from build123d import *

# Parameters (mm, degrees)
SKETCH1_W                    = 1415
SKETCH1_H                    = 88
BASE_FLANGE1_DEPTH           = 4
EDGE_FLANGE1_STRIP_W         = 28
EDGE_FLANGE1_STRIP_H         = 4
EDGE_FLANGE1_STRIP_CUT_DEPTH = 1415
EDGE_FLANGE1_DEPTH           = 1415
EDGE_FLANGE2_STRIP_W         = 28
EDGE_FLANGE2_STRIP_H         = 4
EDGE_FLANGE2_STRIP_CUT_DEPTH = 1415
EDGE_FLANGE2_DEPTH           = 1415
CUT_EXTRUDE1_DEPTH           = 871.900176512
CUT_EXTRUDE1_DEPTH_BACK      = 871.900176512
SKETCH12_R                   = 11
CUT_EXTRUDE2_DEPTH           = 872.093059006
SKETCH16_R                   = 5
CUT_EXTRUDE4_DEPTH           = 10


# Sheet-metal steps are written as plain solids
with BuildPart() as part:
    # Sketch1 → Base-Flange1 (new body)
    with BuildSketch(Plane.XY):
        with Locations((-158.018987342, 44)):
            Rectangle(SKETCH1_W, SKETCH1_H)
    extrude(amount=-BASE_FLANGE1_DEPTH)

    # Edge-Flange1 strip (across the edge) → Edge-Flange1 strip cut (cut)
    with BuildSketch(Plane(origin=(549.481012658, 88, 0), x_dir=(0, -1, 0), z_dir=(-1, 0, 0))):
        with Locations((-4, -2)):
            Rectangle(EDGE_FLANGE1_STRIP_W, EDGE_FLANGE1_STRIP_H)
    extrude(amount=EDGE_FLANGE1_STRIP_CUT_DEPTH, mode=Mode.SUBTRACT)

    # Edge-Flange1 section (across the edge) → Edge-Flange1 (add)
    with BuildSketch(Plane(origin=(549.481012658, 88, 0), x_dir=(0, -1, 0), z_dir=(-1, 0, 0))):
        with BuildLine():
            Line((0, 6), (0, 40))
            Line((0, 40), (4, 40))
            Line((4, 40), (4, 6))
            ThreePointArc((4, 6), (5.757359313, 1.757359313), (10, 0))
            Line((10, 0), (10, -4))
            ThreePointArc((10, -4), (2.928932188, -1.071067812), (0, 6))
        make_face()
    extrude(amount=EDGE_FLANGE1_DEPTH)

    # Edge-Flange2 strip (across the edge) → Edge-Flange2 strip cut (cut)
    with BuildSketch(Plane.YZ.offset(-865.518987342)):
        with Locations((-4, -2)):
            Rectangle(EDGE_FLANGE2_STRIP_W, EDGE_FLANGE2_STRIP_H)
    extrude(amount=EDGE_FLANGE2_STRIP_CUT_DEPTH, mode=Mode.SUBTRACT)

    # Edge-Flange2 section (across the edge) → Edge-Flange2 (add)
    with BuildSketch(Plane.YZ.offset(-865.518987342)):
        with BuildLine():
            Line((0, 6), (0, 40))
            Line((0, 40), (4, 40))
            Line((4, 40), (4, 6))
            ThreePointArc((4, 6), (5.757359313, 1.757359313), (10, 0))
            Line((10, 0), (10, -4))
            ThreePointArc((10, -4), (2.928932188, -1.071067812), (0, 6))
        make_face()
    extrude(amount=EDGE_FLANGE2_DEPTH)

    # Sketch12 → Cut-Extrude1 (cut, two sides: drawn at the far end of the back side and taken through both)
    with BuildSketch(Plane.XZ.offset(-CUT_EXTRUDE1_DEPTH_BACK)):
        with Locations(Location((529.481012658, 20, 0), (0, 0, 270))):
            Circle(SKETCH12_R)
        with Locations(Location((449.481012658, 20, 0), (0, 0, 270))):
            Circle(SKETCH12_R)
    extrude(amount=CUT_EXTRUDE1_DEPTH + CUT_EXTRUDE1_DEPTH_BACK, mode=Mode.SUBTRACT)

    # Sketch13 → Cut-Extrude2 (cut, through all)
    with BuildSketch(Plane(origin=(0, 0, -4), x_dir=(-1, 0, 0), z_dir=(0, 0, -1))):
        with BuildLine():
            Line((850.518987342, 15), (830.518987342, 15))
            ThreePointArc((830.518987342, 15), (825.518987342, 20), (830.518987342, 25))
            Line((830.518987342, 25), (850.518987342, 25))
            ThreePointArc((850.518987342, 25), (855.518987342, 20), (850.518987342, 15))
        make_face()
        with BuildLine():
            Line((750.518987342, 15), (730.518987342, 15))
            ThreePointArc((730.518987342, 15), (725.518987342, 20), (730.518987342, 25))
            Line((730.518987342, 25), (750.518987342, 25))
            ThreePointArc((750.518987342, 25), (755.518987342, 20), (750.518987342, 15))
        make_face()
    extrude(amount=-CUT_EXTRUDE2_DEPTH, mode=Mode.SUBTRACT)

    # Sketch16 → Cut-Extrude4 (cut)
    with BuildSketch(Plane(origin=(0, 0, -4), x_dir=(-1, 0, 0), z_dir=(0, 0, -1))):
        with Locations((509.018987342, 20)):
            Circle(SKETCH16_R)
    extrude(amount=-CUT_EXTRUDE4_DEPTH, mode=Mode.SUBTRACT)


solid = part.part
Design review of the part built by this model. Coordinates are the model's own, in mm. A direction names the side the tool comes from. Coordinates: 2 decimals unless noted, no trailing zeros. Loops run counter-clockwise (first coordinate to the right, second up) from the corner with the lowest first, then second, coordinate; pieces in that order, holes last.
Item 1: Clearance check with flat-ended pins moving along their axes: pin 1 (1.2 mm diameter, centred on x = -841.5, z = -3, fed in from -Y); pin 2 (1.2 mm diameter, centred on x = -839, z = -2.5, fed in from +Y); pin 3 (4.5 mm diameter, centred on x = -737.5, z = -2, fed in from +Y); pin 4 (3 mm diameter, centred on x = -523, z = 31.5, fed in from -Y). State where each tip first meets the part, or that it passes through.
Completed:
pin 1: stops at y = 4.57
pin 2: stops at y = 84.13
pin 3: stops at y = 86.18
pin 4: stops at y = 0
Item 2: Draft analysis for pull direction X (two halves, no side actions). For faces 1 (the cylindrical face through (518.74, 2.03, 22.38)), 2 (the flat face through (-148, 88, 23)), 3 (the flat face through (549.481, 44, -1)), state which applies: pulls with the +X half, pulls with the -X half, needs draft (parallel to the pull), parting line crosses it, or undercut.
Completed:
face 1: undercut
face 2: needs draft
face 3: pulls with the +X half
Item 3: Add section B-B (x = -325). Write out the cut boundary in (y, z).
Completed:
outline: (0, 6) arc R10 ccw to (10, -4) - (78, -4) arc R10 ccw to (88, 6) - (88, 40) - (84, 40) - (84, 6) arc R6 cw to (78, 0) - (10, 0) arc R6 cw to (4, 6) - (4, 40) - (0, 40) - close
Item 4: Add section A-A (z = 20). Write out the cut boundary in (x, y).
Completed:
outline: (-865.52, 0) - (438.48, 0) - (438.48, 4) - (-865.52, 4) - close; (-865.52, 84) - (438.48, 84) - (438.48, 88) - (-865.52, 88) - close; (460.48, 0) - (518.48, 0) - (518.48, 4) - (460.48, 4) - close; (460.48, 84) - (518.48, 84) - (518.48, 88) - (460.48, 88) - close; (540.48, 0) - (549.48, 0) - (549.48, 4) - (540.48, 4) - close; (540.48, 84) - (549.48, 84) - (549.48, 88) - (540.48, 88) - close
Item 5: For faces 4 (the cylindrical face through (518.74, 86.03, 22.38)), 5 (the flat face through (-148, 84, 23)), list the 3-axis set-ups (+Z, -Z, +X, -X, +Y, -Y) from which the entire face can be reached by the end or side of a thin tool; tool diameter is ignored.
Completed:
face 4: +Y, -Y
face 5: +Z, +X, -X
Item 6: Wall thickness on L1, parallel to X at y = 1.5, z = 20; L2, parallel to Y at x = -94, z = 32.5; L3, parallel to Z at x = -456.5, y = 33: over which ranges is each line inside the solid? List them lowest first.
Completed:
L1: x = -865.52 to 438.48, 460.48 to 518.48, 540.48 to 549.48
L2: y = 0 to 4, 84 to 88
L3: z = -4 to 0
Item 7: Add section C-C (y = 47). Write out the cut boundary in (x, z), and give its area (3 significant figures).
Completed:
outline: (-865.52, -4) - (549.48, -4) - (549.48, 0) - (-865.52, 0) - close
area: 5,660 mm2
